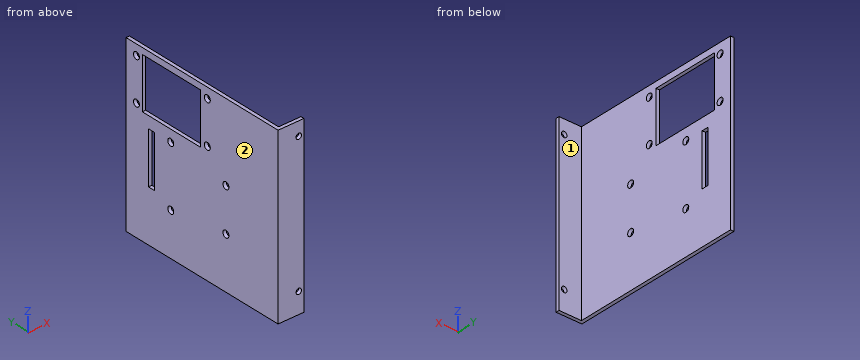
Autodesk Inventor part; units mm, degrees
ref_plane "YZ Plane" through (0, 0, 0) normal (1, 0, 0) x (0, 1, 0)
ref_plane "XZ Plane" through (0, 0, 0) normal (0, 1, 0) x (-1, 0, 0)
ref_plane "XY Plane" through (0, 0, 0) normal (0, 0, 1) x (1, 0, 0)
sketch "草图1" plane through (0, 0, 0) normal (1, 0, 0) x (0, 1, 0)
  line L0 (0, 0) -> (100, 0)
  line L1 (100, 0) -> (100, -100)
  line L2 (100, -100) -> (0, -100)
  line L3 (0, -100) -> (0, 0)
  dimension "d0" = 100
  dimension "d1" = 100
extrude "拉伸1" add sketch "草图1" along normal blind 2
sketch "草图2" plane through (0, 0, -100) normal (0, -1, 0) x (1, 0, 0)
  line L0 (0, 0) -> (0, 100)
  line L1 (0, 100) -> (15, 100)
  line L2 (15, 100) -> (15, 0)
  line L3 (15, 0) -> (0, 0)
  line L4 (0, 0) -> (0, 100)
  dimension "d30" = 15
extrude "拉伸2" add sketch "草图2" along normal blind 2
sketch "草图3" plane through (0, -2, -100) normal (0, -1, 0) x (1, 0, 0)
  circle A0 centre (12, 92) radius 1.6
  line L0 (0, 100) -> (0, 0)
  circle A1 centre (12, 12) radius 1.6
  line L1 (0, 0) -> (15, 0)
  dimension "d6" = 12
  dimension "d7" = 12
  dimension "d8" = 80
  dimension "d9" = 12
  dimension "d12" = 3.2
  dimension "d13" = 3.2
extrude "拉伸3" cut sketch "草图3" against normal blind 2
sketch "草图4" plane through (2, 0, 0) normal (1, 0, 0) x (0, 0, -1)
  line L0 (40, 85) -> (70, 85)
  line L1 (70, 85) -> (70, 81)
  line L2 (70, 81) -> (40, 81)
  line L3 (40, 81) -> (40, 85)
  line L4 (100, 100) -> (0, 100)
  line L5 (0, 100) -> (0, 0)
  circle A0 centre (40, 70) radius 2
  circle A1 centre (75, 70) radius 2
  circle A2 centre (70, 33) radius 2
  circle A3 centre (45, 33) radius 2
  point P0 (40, 83)
  point P1 (70, 83)
  dimension "d14" = 30
  dimension "d15" = 15
  dimension "d16" = 40
  dimension "d17" = 4
  dimension "d18" = 13
  dimension "d19" = 13
  dimension "d20" = 35
  dimension "d21" = 5
  dimension "d22" = 37
  dimension "d23" = 25
  dimension "d24" = 4
  dimension "d25" = 4
  dimension "d26" = 4
  dimension "d27" = 4
extrude "拉伸4" cut sketch "草图4" against normal blind 2
sketch "草图5" plane through (2, 0, 0) normal (1, 0, 0) x (0, 0, -1)
  circle A0 centre (6, 93) radius 2
  circle A1 centre (30.5, 93) radius 2
  circle A2 centre (6, 45.5) radius 2
  line L0 (100, 100) -> (0, 100)
  line L1 (0, 100) -> (0, 0)
  circle A3 centre (30.5, 45.5) radius 2
  dimension "d31" = 4
  dimension "d32" = 4
  dimension "d33" = 24.5
  dimension "d34" = 47.5
  dimension "d35" = 7
  dimension "d36" = 7
  dimension "d37" = 6
  dimension "d38" = 6
  dimension "d39" = 4
  dimension "d40" = 4
sketch "草图6" plane through (2, 0, 0) normal (1, 0, 0) x (0, 0, -1)
  line L0 (3.5741, 89.1195) -> (33.1877, 89.1195)
  line L1 (33.1877, 89.1195) -> (33.1877, 49.9441)
  line L2 (33.1877, 49.9441) -> (3.5741, 49.9441)
  line L3 (3.5741, 49.9441) -> (3.5741, 89.1195)
  point P0 (0, 0)
extrude "拉伸5" cut sketch "草图6" against normal blind 2
extrude "拉伸6" cut sketch "草图5" against normal blind 2
properties part number "板"
Geometry check sheet. Reference: the model listing, model coordinates, mm. Face numbers are marked on the shaded views. A direction names the side the tool comes from. Coordinates: 2 decimals unless noted, no trailing zeros. Order: outer loops, then holes, each group sorted by start corner. A loop starts at its lowest first (then second) coordinate and runs counter-clockwise, first axis right, second up. Notation, with made-up numbers: (62, 45) - (120, 45) arc R19 ccw to (120, 53) - close; hole circle Ø6 at (2.25, 47.5). An arc over 180 degrees is marked (long way). Answer in a Markdown table with one row per item. Add a question column.
1) Cross-section at C-C, the plane y = 66. Record the cut outline in (x, z), then the cut area to 3 significant figures.
2) Gauge pin test, flat ends, axial feed: P1, Ø1, axis at y = 20.5, z = -17, coming from the -X side; P2, Ø3.5, axis at y = 45.5, z = -6, coming from the -X side (3 decimals); P3, Ø6.5, axis at y = 93, z = -6, coming from the +X side; P4, Ø4, axis at x = 9.5, z = -29, coming from the +Y side. Record the tip position at first contact, or that the pin passes through.
3) Set-up check for the marked faces 1 and 2: record each of +Z, -Z, +X, -X, +Y, -Y from which the full face is reachable in a straight line by a thin tool's end or side.
4) Cross-section at A-A, the plane x = 12. Record the cut outline in (y, z).
5) Cross-section at D-D, the plane z = -45. Record the cut outline in (x, y), then the cut area to 3 significant figures.
6) Material ranges on line 1 along Y through (x, z) = (1.35, -45); line 2 along Z through (x, y) = (12, -0.8); line 3 along Y through (x, z) = (13, -49.5), recorded low to high. Write a range as [from, to].
7) Cross-section at B-B, the plane z = -22.5. Record the cut outline in (x, y), then the cut area to 3 significant figures.
Check result:
| question | item | result |
|---|---|---|
| 1 | outline | (0, -100) - (2, -100) - (2, -33.19) - (0, -33.19) - close; (0, -3.57) - (2, -3.57) - (2, 0) - (0, 0) - close |
| 1 | area | 141 mm² |
| 2 | P1 | stops at x = 0 |
| 2 | P2 | passes through |
| 2 | P3 | stops at x = 2 |
| 2 | P4 | stops at y = 0 |
| 3 | face 1 | +Z, -Z, +X, +Y |
| 3 | face 2 | +Z, -Z, -X, +Y, -Y |
| 4 | outline | (-2, -100) - (0, -100) - (0, -89.6) - (-2, -89.6) - close; (-2, -86.4) - (0, -86.4) - (0, -9.6) - (-2, -9.6) - close; (-2, -6.4) - (0, -6.4) - (0, 0) - (-2, 0) - close |
| 5 | outline | (0, -2) - (15, -2) - (15, 0) - (2, 0) - (2, 31) - (0, 31) - close; (0, 35) - (2, 35) - (2, 81) - (0, 81) - close; (0, 85) - (2, 85) - (2, 100) - (0, 100) - close |
| 5 | area | 214 mm² |
| 6 | line 1 | y = [-2, 31], [35, 81], [85, 100] |
| 6 | line 2 | z = [-100, -89.6], [-86.4, -9.6], [-6.4, 0] |
| 6 | line 3 | y = [-2, 0] |
| 7 | outline | (0, -2) - (15, -2) - (15, 0) - (2, 0) - (2, 49.94) - (0, 49.94) - close; (0, 89.12) - (2, 89.12) - (2, 100) - (0, 100) - close |
| 7 | area | 152 mm² |
